Model file for the job. Use its own axes, mm. Give positions to 0.01 mm unless a question says otherwise; leave off trailing zeros. Loops run counter-clockwise (first coordinate to the right, second up) from the corner with the lowest first, then second, coordinate; pieces in that order, holes last. Notation, with made-up numbers: M 83.5,89 L 114.5,89 A17 cw 114.5,111 Z; hole C -13.5,20.25 d3. An arc over 180 degrees is marked long. Answer in a Markdown table with one row per item.
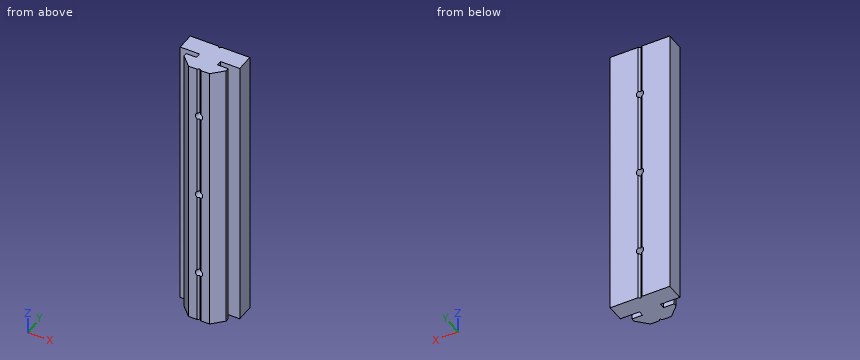
```python
from build123d import *

# Parameters (mm, degrees)
BOSS_EXTRU_1_DEPTH      = 80
ESQUISSE2_R             = 1.05
ENL_V_MAT_EXTRU_1_DEPTH = 82.132607502


with BuildPart() as part:
    # Esquisse1 → Boss.-Extru.1 (new body)
    with BuildSketch(Plane.XY):
        Polygon((0, 10), (0.5, 10.5), (8.5, 10.5), (8.5, 5.5), (3, 5.5), (3, 4), (6, 4), (6, 3), (3, 0), (0.5, 0), (0, 0.5), (-0.5, 0), (-3, 0), (-6, 3), (-6, 4), (-3, 4), (-3, 5.5), (-8.5, 5.5), (-8.5, 10.5), (-0.5, 10.5), align=None)
    extrude(amount=BOSS_EXTRU_1_DEPTH)

    # Esquisse2 → Enlèv. mat.-Extru.1 (cut, through all)
    with BuildSketch(Plane(origin=(0, 10.5, 0), x_dir=(1, 0, 0), z_dir=(0, 1, 0))):
        with Locations(Location((0, -65, 0), (0, 0, 270))):
            Circle(ESQUISSE2_R)
        with Locations(Location((0, -40, 0), (0, 0, 270))):
            Circle(ESQUISSE2_R)
        with Locations(Location((0, -15, 0), (0, 0, 270))):
            Circle(ESQUISSE2_R)
    extrude(amount=-ENL_V_MAT_EXTRU_1_DEPTH, mode=Mode.SUBTRACT)


solid = part.part
```
Q1. Saw through at D-D (x = 7.25). Give the cut face in (y, z).
Reported:
| item | result |
|---|---|
| outline | M 5.5,0 L 10.5,0 L 10.5,80 L 5.5,80 Z |
Q2. Drop flat-ended pins along their axis: pin 1 (1.6 mm diameter, centred on x = -6.5, z = 39.5, fed in from -Y); pin 2 (0.8 mm diameter, centred on y = 3.5, z = 52, fed in from -X); pin 3 (0.8 mm diameter, centred on y = 5, z = 46, fed in from -X). Give the stop position or say it passes through.
Reported:
| item | result |
|---|---|
| pin 1 | y = 2.7 |
| pin 2 | x = -6 |
| pin 3 | x = -3 |
Q3. Probe probe 1 along Z at (x, y) = (0, 4); probe 2 along X at (y, z) = (7, 15); probe 3 along X at (y, z) = (3.25, 65). List the from-to ranges inside material, lowest first.
Reported:
| item | result |
|---|---|
| probe 1 | 0 to 13.95, 16.05 to 38.95, 41.05 to 63.95, 66.05 to 80 |
| probe 2 | -8.5 to -1.05, 1.05 to 8.5 |
| probe 3 | -6 to -1.05, 1.05 to 6 |
Q4. Saw through at C-C (z = 26.5). Give the cut face in (x, y).
Reported:
| item | result |
|---|---|
| outline | M -8.5,5.5 L -3,5.5 L -3,4 L -6,4 L -6,3 L -3,0 L -0.5,0 L 0,0.5 L 0.5,0 L 3,0 L 6,3 L 6,4 L 3,4 L 3,5.5 L 8.5,5.5 L 8.5,10.5 L 0.5,10.5 L 0,10 L -0.5,10.5 L -8.5,10.5 Z |
Q5. Saw through at B-B (z = 40). Give the cut face in (x, y).
Reported:
| item | result |
|---|---|
| outline | M -8.5,5.5 L -3,5.5 L -3,4 L -6,4 L -6,3 L -3,0 L -1.05,0 L -1.05,10.5 L -8.5,10.5 Z; M 1.05,0 L 3,0 L 6,3 L 6,4 L 3,4 L 3,5.5 L 8.5,5.5 L 8.5,10.5 L 1.05,10.5 Z |
Q6. Saw through at A-A (y = 2). Give the cut face in (x, z).
Reported:
| item | result |
|---|---|
| outline | M -5,0 L 5,0 L 5,80 L -5,80 Z; hole C 0,15 d2.1; hole C 0,40 d2.1; hole C 0,65 d2.1 |
